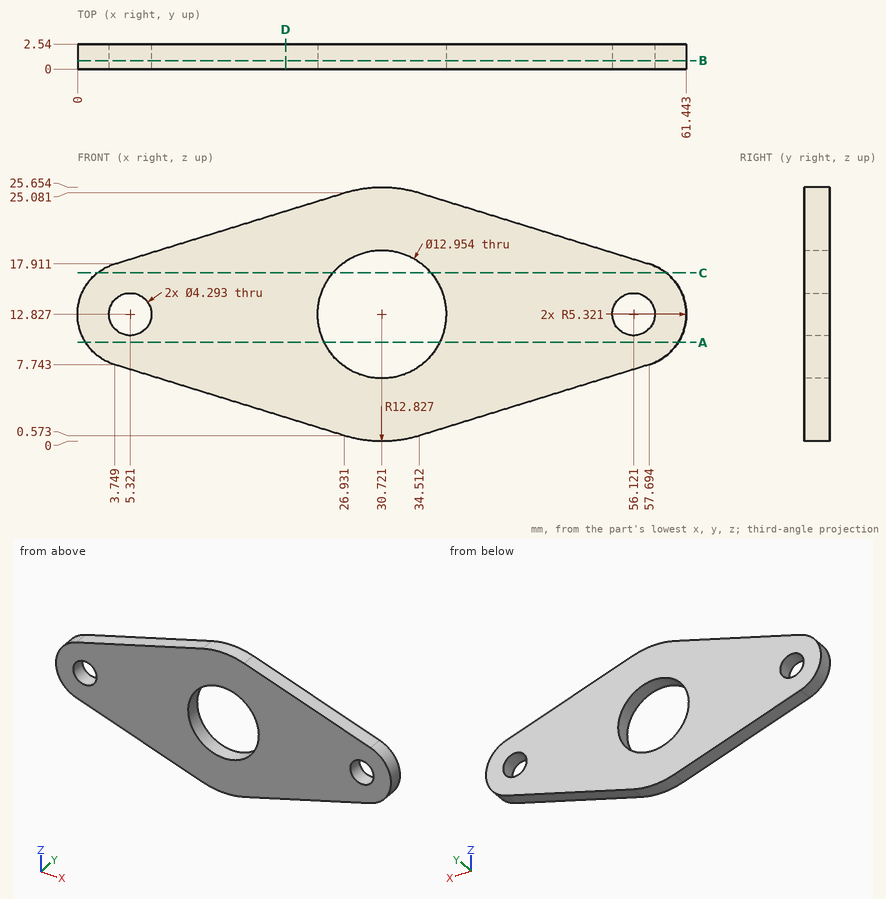
Can you work these out from the drawing? Everything is in mm from the part's minimum corner. Coordinates: 2 decimals unless noted, no trailing zeros. Loops run counter-clockwise (first coordinate to the right, second up) from the corner with the lowest first, then second, coordinate; pieces in that order, holes last.
1) Imagine slicing it at B-B (y = 0.85). List the corners of the cut face in (x, z) for me, and give its area (3 significant figures).
Reported:
outline: (3.75, 7.74) - (26.93, 0.57) arc R12.83 ccw to (34.51, 0.57) - (57.69, 7.74) arc R5.32 ccw to (57.69, 17.91) - (34.51, 25.08) arc R12.83 ccw to (26.93, 25.08) - (3.75, 17.91) arc R5.32 ccw to start; hole circle Ø4.29 at (5.32, 12.83); hole circle Ø12.95 at (30.72, 12.83); hole circle Ø4.29 at (56.12, 12.83)
area: 891 mm2
2) Imagine slicing it at D-D (x = 21). List the corners of the cut face in (y, z) for me.
Reported:
outline: (0, 2.41) - (2.54, 2.41) - (2.54, 23.25) - (0, 23.25) - close
3) Imagine slicing it at C-C (z = 17). List the corners of the cut face in (x, y) for me (1 decimal).
Reported:
outline: (2, 0) - (25.8, 0) - (25.8, 2.5) - (2, 2.5) - close; (35.7, 0) - (59.4, 0) - (59.4, 2.5) - (35.7, 2.5) - close
4) Will this pin go through, and if not, where does the flat tip stop? pin 1 Ø1.5 at (x, y) = (13, 2) entering from +Z.
Reported:
pin 1: stops at z = 21
5) Please list where these lines run through material, in increasing order: line 1 along X through (y, z) = (0.3, 12.5); line 2 along X through (y, z) = (1.35, 16.5) (1 decimal); line 3 along X through (y, z) = (2.1, 8.5) (1 decimal).
Reported:
line 1: x = 0.01 to 3.2, 7.44 to 24.25, 37.19 to 54, 58.24 to 61.43
line 2: x = 1.5 to 25.4, 36.1 to 60
line 3: x = 2.2 to 25.9, 35.5 to 59.2
6) Imagine slicing it at A-A (z = 10). List the corners of the cut face in (x, y) for me, and give its area (3 significant figures).
Reported:
outline: (0.81, 0) - (24.89, 0) - (24.89, 2.54) - (0.81, 2.54) - close; (36.55, 0) - (60.63, 0) - (60.63, 2.54) - (36.55, 2.54) - close
area: 122 mm2
